Design review of the part shown in the three views and the two pictorial views. Dimensions are in mm from the part's minimum x, y and z. A direction names the side the tool comes from. Give positions to 0.01 mm unless a question says otherwise; leave off trailing zeros. Loops run counter-clockwise (first coordinate to the right, second up) from the corner with the lowest first, then second, coordinate; pieces in that order, holes last. Notation, with made-up numbers: (29.25, -31.75) - (35.25, -31.75) arc R32 cw to (35.25, 1.25) - close; hole circle Ø5 at (88.25, -35.5). An arc over 180 degrees is marked (long way). Return JSON: item names as keys, results as strings. Group by question number.
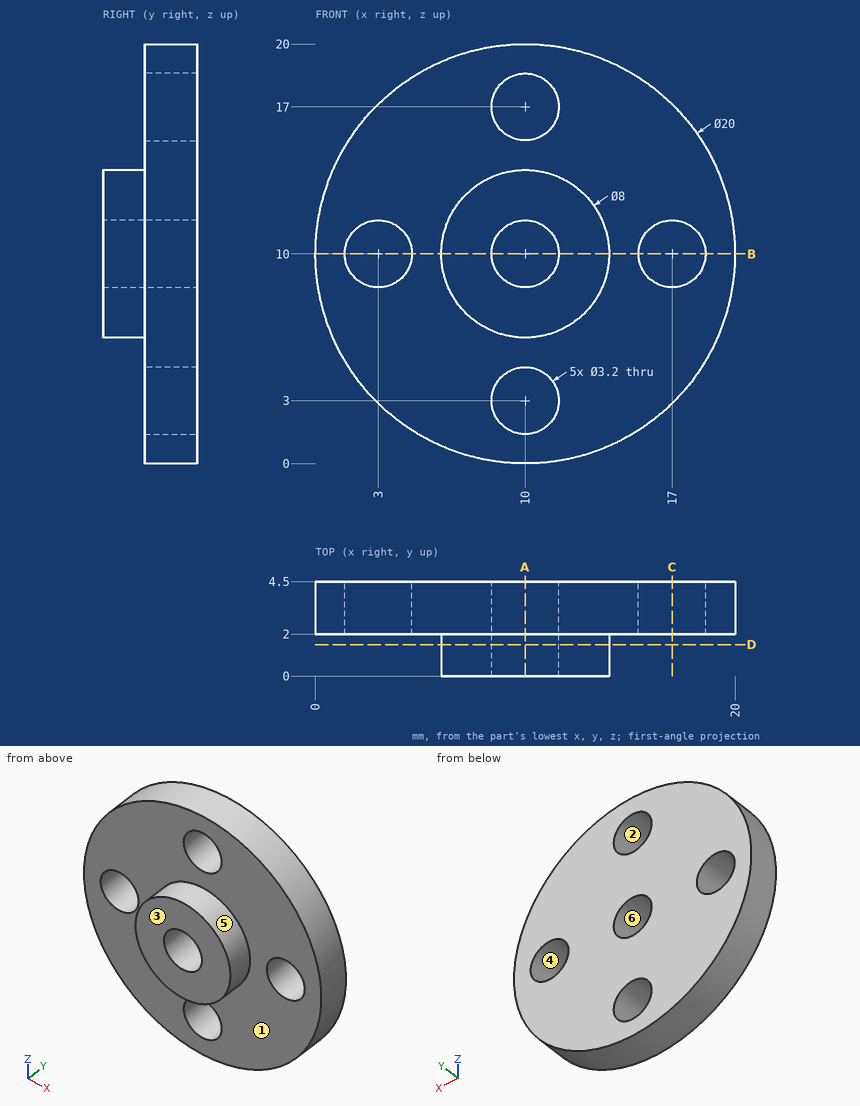
Item 1: For P1, Ø2, axis at x = 16.5, z = 15, coming from the -Y side, flat-tipped, find the tip position at first contact; note if it passes through.
Item 2: Take a section at A-A (x = 10). State the section outline as (y, z) points.
Item 3: Take a section at B-B (z = 10). State the section outline as (x, y) points, then the cut area to 3 significant figures.
Item 4: Tool access review of the marked faces 1 and 2: name each direction out of +Z, -Z, +X, -X, +Y, -Y from which nothing blocks a thin tool from reaching the whole face with its end or side.
Item 5: Mouldability with a two-part tool opening along Z and no side actions: class the marked faces 3, 4, 5 and 6 as +Z half, -Z half, draft (parallel to the pull), parting line (faces both ways), or undercut.
Item 6: For L1, parallel to X at y = 2.7, z = 10; L2, parallel to Z at x = 10.25, y = 1.4; L3, parallel to Y at x = 10.25, z = 18.75, list the stretches that pass through material, from the lowest coordinate up. Write a range as from..to.
Item 7: Take a section at C-C (x = 17). State the section outline as (y, z) points.
Item 8: Take a section at D-D (y = 1.5). State the section outline as (x, z) points.
Check sheet entries:
{
 "1": {"P1": "stops at y = 2"},
 "2": {"outline": "(0, 6) - (2, 6) - (2, 4.6) - (4.5, 4.6) - (4.5, 8.4) - (0, 8.4) - close; (0, 11.6) - (4.5, 11.6) - (4.5, 15.4) - (2, 15.4) - (2, 14) - (0, 14) - close; (2, 0) - (4.5, 0) - (4.5, 1.4) - (2, 1.4) - close; (2, 18.6) - (4.5, 18.6) - (4.5, 20) - (2, 20) - close"},
 "3": {"outline": "(0, 2) - (1.4, 2) - (1.4, 4.5) - (0, 4.5) - close; (4.6, 2) - (6, 2) - (6, 0) - (8.4, 0) - (8.4, 4.5) - (4.6, 4.5) - close; (11.6, 0) - (14, 0) - (14, 2) - (15.4, 2) - (15.4, 4.5) - (11.6, 4.5) - close; (18.6, 2) - (20, 2) - (20, 4.5) - (18.6, 4.5) - close", "area": "35.6 mm^2"},
 "4": {"face 1": "-Y", "face 2": "+Y, -Y"},
 "5": {"face 3": "draft", "face 4": "undercut", "face 5": "parting line", "face 6": "undercut"},
 "6": {"L1": "x = 0..1.4, 4.6..8.4, 11.6..15.4, 18.6..20", "L2": "z = 6.01..8.42, 11.58..13.99", "L3": "y = 2..4.5"},
 "7": {"outline": "(2, 2.86) - (4.5, 2.86) - (4.5, 8.4) - (2, 8.4) - close; (2, 11.6) - (4.5, 11.6) - (4.5, 17.14) - (2, 17.14) - close"},
 "8": {"outline": "circle Ø8 at (10, 10); hole circle Ø3.2 at (10, 10)"}
}
